from build123d import *

# Parameters (mm, degrees)
SKETCH_1_W          = 2.65
SKETCH_1_H          = 5.9
EXTRUDE_3_DEPTH     = 3
EXTRUDE_3_2_DEPTH   = 3
SKETCH_1_3_W        = 5
SKETCH_1_3_H        = 5.9
SKETCH_1_3_R        = 2
EXTRUDE_4_DEPTH     = 5
CUT_EXTRUDE_1_DEPTH = 10.2915284


with BuildPart() as part:
    # Sketch 1 → Extrude 3 (new body)
    with BuildSketch(Plane(origin=(0, 0, 0), x_dir=(1, 0, 0), z_dir=(0, 1, 0))):
        with Locations((-3.825, 0)):
            Rectangle(SKETCH_1_W, SKETCH_1_H)
    extrude(amount=EXTRUDE_3_DEPTH)



with BuildPart() as body_2:
    # Sketch 1 → Extrude 3 2 (new body)
    with BuildSketch(Plane(origin=(0, 0, 0), x_dir=(1, 0, 0), z_dir=(0, 1, 0))):
        with Locations((3.825, 0)):
            Rectangle(SKETCH_1_W, SKETCH_1_H)
    extrude(amount=EXTRUDE_3_2_DEPTH)


with BuildPart() as part_1:
    add(part.part)

    add(body_2.part)  # Extrude 4 merges body 2
    # Sketch 1_3 → Extrude 4 (add)
    with BuildSketch(Plane(origin=(0, 0, 0), x_dir=(1, 0, 0), z_dir=(0, 1, 0))):
        Rectangle(SKETCH_1_3_W, SKETCH_1_3_H)
        with Locations(Location((0, 0, 0), (0, 0, 270))):
            Circle(SKETCH_1_3_R, mode=Mode.SUBTRACT)
    extrude(amount=EXTRUDE_4_DEPTH)

    # Sketch 2 → Cut-Extrude 1 (cut, through all)
    with BuildSketch(Plane.XY.offset(2.95)):
        Polygon((-5.15, 1.5), (-3.65, 0), (-5.15, 0), align=None)
        Polygon((5.15, 1.5), (3.65, 0), (5.15, 0), align=None)
    extrude(amount=-CUT_EXTRUDE_1_DEPTH, mode=Mode.SUBTRACT)


solid = part_1.part
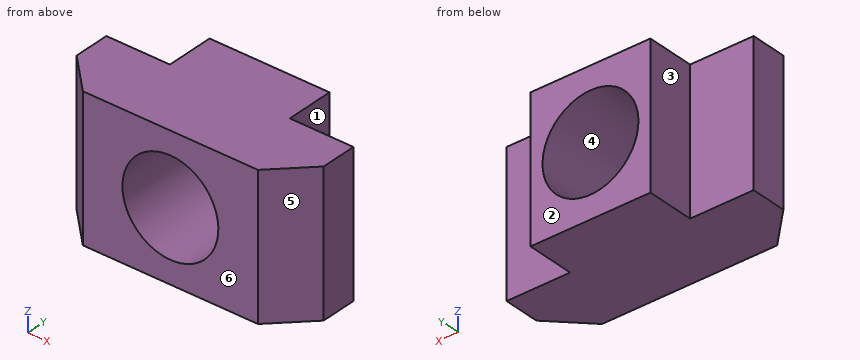
Design review of the part built by this model. Coordinates are the model's own, in mm. Face numbers are marked on the shaded views. A direction names the side the tool comes from. Give positions to 0.01 mm unless a question says otherwise; leave off trailing zeros. Order: outer loops, then holes, each group sorted by start corner. A loop starts at its lowest first (then second) coordinate and runs counter-clockwise, first axis right, second up. Notation, with made-up numbers: (-39.75, 56.5) - (-10.75, 56.5) arc R22 ccw to (-10.75, 76.5) - close; hole circle Ø10 at (-25, -5). An arc over 180 degrees is marked (long way). Write item = value, one per line. Start each with the question number.
Q1. To check wall thickness, follow L1, parallel to X at y = 2.2, z = 0; L2, parallel to X at y = 3.45, z = 0; L3, parallel to Y at x = -3.5, z = -2.3. State the ranges of each line that lie inside material, in increasing order. Write a range as from..to.
Q2. Clearance check with flat-ended pins moving along their axes: pin 1 Ø1 at (y, z) = (4, 0) entering from +X; pin 2 Ø1.6 at (y, z) = (4, 1.5) entering from -X. State where each tip first meets the part, or that it passes through.
Q3. We need section B-B on z = 0. State the section outline as (x, y) points.
Q4. We need section C-C on y = 2.05. State the section outline as (x, z) points, plus the area to 3 significant figures.
Q5. We need section D-D on z = 2.55. State the section outline as (x, y) points.
Q6. Mouldability with a two-part tool opening along X and no side actions: class the marked faces 4, 5 and 6 as released by +X, released by -X, zero draft, split by the parting line, or undercut.
Q7. We need section A-A on x = 0. State the section outline as (y, z) points, plus the area to 3 significant figures.
Q8. Tool access review of the marked faces 1, 2 and 3: name each direction out of +Z, -Z, +X, -X, +Y, -Y from which nothing blocks a thin tool from reaching the whole face with its end or side.
Working result:
q1.L1 = -5.15..-2, 2..5.15
q1.L2 = -2.5..-2, 2..2.5
q1.L3 = 0..3
q2.pin_1 = 2.5
q2.pin_2 = -2.5
q3.outline = (-5.15, 1.5) - (-3.65, 0) - (-2, 0) - (-2, 5) - (-2.5, 5) - (-2.5, 3) - (-5.15, 3) - close; (2, 0) - (3.65, 0) - (5.15, 1.5) - (5.15, 3) - (2.5, 3) - (2.5, 5) - (2, 5) - close
q4.outline = (-5.15, -2.95) - (5.15, -2.95) - (5.15, 2.95) - (-5.15, 2.95) - close; hole circle Ø4 at (0, 0)
q4.area = 48.2 mm²
q5.outline = (-5.15, 1.5) - (-3.65, 0) - (3.65, 0) - (5.15, 1.5) - (5.15, 3) - (2.5, 3) - (2.5, 5) - (-2.5, 5) - (-2.5, 3) - (-5.15, 3) - close
q6.face_4 = undercut
q6.face_5 = released by +X
q6.face_6 = zero draft
q7.outline = (0, -2.95) - (5, -2.95) - (5, -2) - (0, -2) - close; (0, 2) - (5, 2) - (5, 2.95) - (0, 2.95) - close
q7.area = 9.50 mm²
q8.face_1 = +Z, -Z, +X, +Y
q8.face_2 = +Z, -Z, +X, -X, +Y
q8.face_3 = +Z, -Z, -X, +Y
